Geometry: final body of the model. Coordinates: model frame, mm. Round coordinates to 2 decimals unless told otherwise and drop trailing zeros. Write each loop counter-clockwise with the first axis right and the second up, starting at its lowest first coordinate (ties: lowest second). Pieces come first, ordered by that corner, then holes. Notation, with made-up numbers: M -26.75,0.25 L 16.25,0.25 A30 ccw 16.25,38.25 Z; hole C -6,24 d10. An arc over 180 degrees is marked long. Use one line per item in the form item = value. Start each with the question number.
Item 1: Pull-direction query (X, two-part tool) for faces 1 (the flat face through (2, 40.3, -0.5)), 2 (the cylindrical face through (6.751, 34.538, -0.493)), 3 (the cylindrical face through (27.87, 31.69, -0.49)), 4 (the flat face through (30, 12, -1)); classes: pulls with the +X half, pulls with the -X half, needs draft (parallel to the pull), parting line crosses it, or undercut.
Item 2: Ray query, probe 1 along Y at (x, z) = (36.5, -0.7); probe 2 along X at (y, z) = (5, -0.5); probe 3 along Y at (x, z) = (21.15, -0.4). Return the intervals inside material, ascending.
Item 3: Section query D-D (x = 6). Return loops of the section in (y, z).
Item 4: Pin query (flat end, axial travel): pin 1 Ø2 at (x, y) = (6.5, 15.5) entering from +Z; pin 2 Ø4.5 at (x, y) = (5.655, 36.645) entering from +Z. Return the tip coordinate at first contact, or that it passes through.
Item 5: Section query A-A (y = 21.15). Return loops of the section in (x, z).
Item 6: Section query C-C (z = -0.65). Return loops of the section in (x, y) (3 decimals), and give its area (3 significant figures).
from build123d import *

# Parameters (mm, degrees)
F0_R     = 2.375
F0_R_2   = 12.5
F1_DEPTH = 1


with BuildPart() as f1:
    # F0 (on Top) → F1 (new body)
    with BuildSketch(Plane.XY):
        Polygon((0, 4), (4, 0), (38.3, 0), (42.3, 4), (42.3, 38.3), (38.3, 42.3), (4, 42.3), (0, 38.3), align=None)
        with Locations((5.655, 5.655)):
            Circle(F0_R, mode=Mode.SUBTRACT)
        with Locations((36.645, 5.655)):
            Circle(F0_R, mode=Mode.SUBTRACT)
        with Locations((5.655, 36.645)):
            Circle(F0_R, mode=Mode.SUBTRACT)
        with Locations((21.15, 21.15)):
            Circle(F0_R_2, mode=Mode.SUBTRACT)
        with Locations((36.645, 36.645)):
            Circle(F0_R, mode=Mode.SUBTRACT)
    extrude(amount=-F1_DEPTH)


solid = f1.part
Working result:
q1.face_1 = pulls with the -X half
q1.face_2 = undercut
q1.face_3 = undercut
q1.face_4 = needs draft
q2.probe_1 = 0 to 3.28, 8.03 to 34.27, 39.02 to 42.3
q2.probe_2 = 0 to 3.37, 7.94 to 34.36, 38.93 to 42.3
q2.probe_3 = 0 to 8.65, 33.65 to 42.3
q3.outline = M 0,-1 L 3.31,-1 L 3.31,0 L 0,0 Z; M 8,-1 L 34.3,-1 L 34.3,0 L 8,0 Z; M 38.99,-1 L 42.3,-1 L 42.3,0 L 38.99,0 Z
q4.pin_1 = 0
q4.pin_2 = through
q5.outline = M 0,-1 L 8.65,-1 L 8.65,0 L 0,0 Z; M 33.65,-1 L 42.3,-1 L 42.3,0 L 33.65,0 Z
q6.outline = M 0,4 L 4,0 L 38.3,0 L 42.3,4 L 42.3,38.3 L 38.3,42.3 L 4,42.3 L 0,38.3 Z; hole C 5.655,5.655 d4.75; hole C 5.655,36.645 d4.75; hole C 21.15,21.15 d25; hole C 36.645,5.655 d4.75; hole C 36.645,36.645 d4.75
q6.area = 1,200 mm²
